from build123d import *

# Parameters (mm, degrees)
SKETCH1_R                                            = 1.7272
BOSS_EXTRUDE1_DEPTH                                  = 3.175
FILLET2_R                                            = 8.4836
SKETCH2_R                                            = 3.175
BOSS_EXTRUDE2_DEPTH                                  = 3.175
CSK_FOR_M2_5_CROSS_COUNTERSUNK_HEAD_SCRE_D           = 3.1
CSK_FOR_M2_5_CROSS_COUNTERSUNK_HEAD_SCRE_CSINK_D     = 5
CSK_FOR_M2_5_CROSS_COUNTERSUNK_HEAD_SCRE_CSINK_ANGLE = 92
CSK_FOR_M2_5_CROSS_COUNTERSUNK_HEAD_2_D              = 3.1
CSK_FOR_M2_5_CROSS_COUNTERSUNK_HEAD_2_CSINK_D        = 5
CSK_FOR_M2_5_CROSS_COUNTERSUNK_HEAD_2_CSINK_ANGLE    = 92


with BuildPart() as part:
    # Sketch1 → Boss-Extrude1 (new body)
    with BuildSketch(Plane(origin=(0, 0, 0), x_dir=(1, 0, 0), z_dir=(0, 1, 0))):
        with BuildLine():
            Line((-8.4836, 101.245190162), (-8.4836, 109.728790162))
            ThreePointArc((-8.4836, 109.728790162), (0, 118.212390162), (8.4836, 109.728790162))
            Line((8.4836, 109.728790162), (8.4836, 101.245190162))
            ThreePointArc((8.4836, 101.245190162), (71.842048969, 71.842048969), (101.245190162, 8.4836))
            Line((101.245190162, 8.4836), (109.728790162, 8.4836))
            ThreePointArc((109.728790162, 8.4836), (118.212390162, 0), (109.728790162, -8.4836))
            Line((109.728790162, -8.4836), (101.245190162, -8.4836))
            ThreePointArc((101.245190162, -8.4836), (71.842048969, -71.842048969), (8.4836, -101.245190162))
            Line((8.4836, -101.245190162), (8.4836, -109.728790162))
            ThreePointArc((8.4836, -109.728790162), (0, -118.212390162), (-8.4836, -109.728790162))
            Line((-8.4836, -109.728790162), (-8.4836, -101.245190162))
            ThreePointArc((-8.4836, -101.245190162), (-71.842048969, -71.842048969), (-101.245190162, -8.4836))
            Line((-101.245190162, -8.4836), (-109.728790162, -8.4836))
            ThreePointArc((-109.728790162, -8.4836), (-118.212390162, 0), (-109.728790162, 8.4836))
            Line((-109.728790162, 8.4836), (-101.245190162, 8.4836))
            ThreePointArc((-101.245190162, 8.4836), (-71.842048969, 71.842048969), (-8.4836, 101.245190162))
        make_face()
        with Locations(Location((0, 109.728790162, 0), (0, 0, 270))):
            Circle(SKETCH1_R, mode=Mode.SUBTRACT)
        with Locations(Location((109.728790162, 0, 0), (0, 0, 270))):
            Circle(SKETCH1_R, mode=Mode.SUBTRACT)
        with Locations(Location((0, -109.728790162, 0), (0, 0, 270))):
            Circle(SKETCH1_R, mode=Mode.SUBTRACT)
        with Locations(Location((-109.728790163, 0, 0), (0, 0, 270))):
            Circle(SKETCH1_R, mode=Mode.SUBTRACT)
    extrude(amount=BOSS_EXTRUDE1_DEPTH)

    # Fillet2
    fillet2_edges = [part.edges().sort_by_distance(p)[0] for p in [
        (8.4836, 1.5875, -101.245190162),
        (101.245190162, 1.5875, -8.4836),
        (101.245190162, 1.5875, 8.4836),
        (8.4836, 1.5875, 101.245190162),
        (-8.4836, 1.5875, 101.245190162),
        (-101.245190162, 1.5875, 8.4836),
        (-101.245190162, 1.5875, -8.4836),
        (-8.4836, 1.5875, -101.245190162),
    ]]
    fillet(fillet2_edges, radius=FILLET2_R)

    # Sketch2 → Boss-Extrude2 (add)
    with BuildSketch(Plane(origin=(0, 3.175, 0), x_dir=(1, 0, 0), z_dir=(0, 1, 0))):
        with Locations(Location((-37.514063478, -74.985936522, 0), (0, 0, 270))):
            Circle(SKETCH2_R)
        with Locations(Location((-37.514063478, -16.985936522, 0), (0, 0, 270))):
            Circle(SKETCH2_R)
        with Locations(Location((11.485936522, -74.985936522, 0), (0, 0, 90))):
            Circle(SKETCH2_R)
        with Locations(Location((11.485936522, -16.985936522, 0), (0, 0, 90))):
            Circle(SKETCH2_R)
    extrude(amount=BOSS_EXTRUDE2_DEPTH)

    # CSK for M2.5 Cross Countersunk Head Scre (through all)
    with Locations(Plane(origin=(0, 0, 0), x_dir=(-1, 0, 0), z_dir=(0, -1, 0))):
        with Locations((-11.485936522, -16.985936522), (37.514063478, -16.985936522), (37.514063478, -74.985936522), (-11.485936522, -74.985936522)):
            CounterSinkHole(CSK_FOR_M2_5_CROSS_COUNTERSUNK_HEAD_SCRE_D / 2, CSK_FOR_M2_5_CROSS_COUNTERSUNK_HEAD_SCRE_CSINK_D / 2, counter_sink_angle=CSK_FOR_M2_5_CROSS_COUNTERSUNK_HEAD_SCRE_CSINK_ANGLE)

    # CSK for M2.5 Cross Countersunk Head  2 (through all)
    with Locations(Plane(origin=(0, 0, 0), x_dir=(-1, 0, 0), z_dir=(0, -1, 0))):
        with Locations((0, 92.075), (0, -92.075), (92.075, 0), (-92.075, 0)):
            CounterSinkHole(CSK_FOR_M2_5_CROSS_COUNTERSUNK_HEAD_2_D / 2, CSK_FOR_M2_5_CROSS_COUNTERSUNK_HEAD_2_CSINK_D / 2, counter_sink_angle=CSK_FOR_M2_5_CROSS_COUNTERSUNK_HEAD_2_CSINK_ANGLE)


solid = part.part
Work out the finished part from the listing and answer in its coordinate system (mm). A direction names the side the tool comes from. Coordinates: 2 decimals unless noted, no trailing zeros. Write each loop counter-clockwise with the first axis right and the second up, starting at its lowest first coordinate (ties: lowest second). Pieces come first, ordered by that corner, then holes. Notation, with made-up numbers: M 45.5,73.25 L 87.5,73.25 A27 ccw 87.5,108.25 Z; hole C -25.5,-18.5 d11. An arc over 180 degrees is marked long. Write item = value, one per line.
1. Determine the mould class of faces 1 (the face through (10.53, 4.74, 71.96)), 2 (the face through (0.19, 1.57, 118.21)), 3 (the face through (-0.19, 1.57, -118.21)) for opening direction Z: released by +Z, released by -Z, zero draft, split by the parting line, or undercut.
Solution:
face_1 = undercut
face_2 = released by +Z
face_3 = released by -Z
2. Straight lines are drawn through the part: line 1 (Y direction, x = -76.5, z = -10) (3 decimals); line 2 (Z direction, x = 56, y = 0.5); line 3 (X direction, y = 0.75, z = 45). For each, find the intervals that lie inside material, in ascending order. Write a range as from..to.
Solution:
line_1 = 0..3.175
line_2 = -84.77..84.77
line_3 = -91.09..91.09
3. The part is cut by section B-B (z = 66.5). Determine the outline of the cut face in (x, y) (3 decimals).
Solution:
outline = M -76.813,0 L 76.813,0 L 76.813,3.175 L -76.813,3.175 Z
4. The part is cut by section C-C (x = -84). Determine the outline of the cut face in (y, z) (3 decimals), then the cut area to 3 significant figures.
Solution:
outline = M 0,-57.154 L 3.175,-57.154 L 3.175,57.154 L 0,57.154 Z
area = 363 mm2
5. The part is cut by section A-A (y = 4.75). Determine the outline of the cut face in (x, z) (3 decimals), then the cut area to 3 significant figures.
Solution:
outline = C -37.514,16.986 d6.35; C -37.514,74.986 d6.35; C 11.486,16.986 d6.35; C 11.486,74.986 d6.35; hole C -37.514,16.986 d3.1; hole C -37.514,74.986 d3.1; hole C 11.486,16.986 d3.1; hole C 11.486,74.986 d3.1
area = 96.5 mm2
6. Flat-ended cylindrical pins translate along their axes: pin 1 (3 mm diameter, centred on x = 109.73, z = 0, fed in from -Y); pin 2 (3.5 mm diameter, centred on x = -37.51, z = 74.99, fed in from -Y); pin 3 (4.5 mm diameter, centred on x = -109.73, z = 0, fed in from -Y); pin 4 (0.5 mm diameter, centred on y = 1, z = -109, fed in from +X). Find the tip coordinate at first contact, or state that the pin passes through.
Solution:
pin_1 = through
pin_2 = 0.72
pin_3 = 0
pin_4 = 8.48
7. For faces 4 (the face through (-36.56, 4.74, 78.014)), 5 (the face through (2, 0, -2)), determine the directions among +Z, -Z, +X, -X, +Y, -Y from which every point of the face is accessible in a straight line to the end or side of a thin tool.
Solution:
face_4 = +Y
face_5 = +Z, -Z, +X, -X, -Y
